Part model, mm, in its own coordinate system. Give positions to 0.01 mm unless a question says otherwise; leave off trailing zeros. Order: outer loops, then holes, each group sorted by start corner. A loop starts at its lowest first (then second) coordinate and runs counter-clockwise, first axis right, second up. Notation, with made-up numbers: (-3, -30.5) - (3, -30.5) arc R21 cw to (3, -4.5) - close; hole circle Ø11 at (-33, 61). An arc over 180 degrees is marked (long way). One line per item, written item: value.
```python
from build123d import *

# Parameters (mm, degrees)
SKETCH_1_R               = 10
SKETCH_1_R_2             = 3.25
EXTRUDE_1_DEPTH          = 15
SKETCH_2_R               = 1.25
CUT_EXTRUDE_1_DEPTH      = 15
PATTERN_CIRCULAR_1_COUNT = 4
CHAMFER_1_SIZE           = 0.5


with BuildPart() as part:
    # 草图1 → 凸台-拉伸1 (new body)
    with BuildSketch(Plane(origin=(0, 0, 0), x_dir=(1, 0, 0), z_dir=(0, 1, 0))):
        with Locations(Location((0, 0, 0), (0, 0, 270))):
            Circle(SKETCH_1_R)
        with Locations(Location((0, 0, 0), (0, 0, 270))):
            Circle(SKETCH_1_R_2, mode=Mode.SUBTRACT)
    extrude(amount=EXTRUDE_1_DEPTH)

    # 草图2 → 切除-拉伸1 (cut)
    with BuildSketch(Plane(origin=(0, 15, 0), x_dir=(1, 0, 0), z_dir=(0, 1, 0))):
        with Locations(Location((-6.5, 0, 0), (0, 0, 270))):
            Circle(SKETCH_2_R)
    cut_extrude_1 = extrude(amount=-CUT_EXTRUDE_1_DEPTH, mode=Mode.SUBTRACT)

    # 阵列(圆周)1: 切除-拉伸1 ×4 about axis
    pattern_circular_1_axis = Axis((0, 0, 0), (0, 1, 0))
    for i in range(1, PATTERN_CIRCULAR_1_COUNT):
        add(cut_extrude_1.rotate(pattern_circular_1_axis, i * 360 / PATTERN_CIRCULAR_1_COUNT), mode=Mode.SUBTRACT)

    # 倒角1
    chamfer_1_edges = [part.edges().sort_by_distance(p)[0] for p in [
        (-6.5, 0, -1.25),
        (-6.5, 15, -1.25),
        (1.25, 0, -6.5),
        (1.25, 15, -6.5),
        (0, 0, -10),
        (6.5, 0, 1.25),
        (6.5, 15, 1.25),
        (-1.25, 0, 6.5),
        (-1.25, 15, 6.5),
        (0, 15, -10),
        (0, 0, -3.25),
        (0, 15, -3.25),
    ]]
    chamfer(chamfer_1_edges, length=CHAMFER_1_SIZE)


solid = part.part
```
1) Cut at A-A, the plane x = 0. Give the number of separate pieces and of enclosed holes in the cut face, then the cut area to 4 significant figures.
Outcome:
separate pieces: 4
enclosed holes: 0
area: 125.5 mm^2
2) Pin check, flat tips, straight feed: pin 1 (4 mm diameter, centred on x = 0, z = 6.5, fed in from -Y); pin 2 (6 mm diameter, centred on x = 0, z = 0, fed in from +Y) (3 decimals); pin 3 (2 mm diameter, centred on y = 12.5, z = 6.5, fed in from +X); pin 4 (6 mm diameter, centred on x = -5, y = 1.5, fed in from -Z). Stop position of each tip, or through.
Outcome:
pin 1: stops at y = 0
pin 2: passes through
pin 3: stops at x = 8.35
pin 4: stops at z = -9.8
3) Mould opens along Z. For faces 1 (the flat face through (0, 15, 4)), 2 (the cylindrical face through (-7.72, 7.6, -0.27)), 3 (the cylindrical face through (-1.978, 7.402, -2.579)), 4 (the cylindrical face through (-9.76, 7.4, -2.17)) say: released by +Z, released by -Z, zero draft, split by the parting line, or undercut.
Outcome:
face 1: zero draft
face 2: undercut
face 3: undercut
face 4: split by the parting line
4) Drill centre lines: line 1 along X through (y, z) = (10.75, 0); line 2 along Z through (x, y) = (-0.75, 4.25); line 3 along Z through (x, y) = (1, 1.5). Where is each one in solid material? Low to high. Write a range as from..to.
Outcome:
line 1: x = -10..-7.75, -5.25..-3.25, 3.25..5.25, 7.75..10
line 2: z = -9.97..-7.5, -5.5..-3.16, 3.16..5.5, 7.5..9.97
line 3: z = -9.95..-7.25, -5.75..-3.09, 3.09..5.75, 7.25..9.95
5) Cut at C-C, the plane y = 3. Give the cut face in (x, z), then the cut area to 3 significant figures.
Outcome:
outline: circle Ø20 at (0, 0); hole circle Ø2.5 at (-6.5, 0); hole circle Ø6.5 at (0, 0); hole circle Ø2.5 at (0, -6.5); hole circle Ø2.5 at (0, 6.5); hole circle Ø2.5 at (6.5, 0)
area: 261 mm^2
